Check sheet for the modelled part. Datum: model origin and axes. Units: mm. A direction names the side the tool comes from. Coordinates: 2 decimals unless noted, no trailing zeros. Loops run counter-clockwise (first coordinate to the right, second up) from the corner with the lowest first, then second, coordinate; pieces in that order, holes last.
```python
from build123d import *

# Parameters (mm, degrees)
BOSS_EXTRUDE9_DEPTH      = 3.5
BOSS_EXTRUDE9_DEPTH_BACK = 4
SKETCH16_W               = 8
SKETCH16_H               = 3.5
BOSS_EXTRUDE11_DEPTH     = 8
CHAMFER2_SIZE            = 1.5
CUT_EXTRUDE1_DEPTH       = 40.150823276
CUT_EXTRUDE1_DEPTH_BACK  = 40.150823276
SKETCH17_R               = 2.12


with BuildPart() as part:
    # Sketch14 → Boss-Extrude9 (new, two sides: drawn at the far end of the back side and taken through both)
    with BuildSketch(Plane(origin=(0, 0, 0), x_dir=(1, 0, 0), z_dir=(0, 1, 0)).offset(-BOSS_EXTRUDE9_DEPTH_BACK)):
        with BuildLine():
            Line((-4.172171186, -29.619968889), (7.827828814, -29.619968889))
            Line((7.827828814, -29.619968889), (7.827828814, -20.619968889))
            ThreePointArc((7.827828814, -20.619968889), (1.827828814, -14.619968889), (-4.172171186, -20.619968889))
            Line((-4.172171186, -20.619968889), (-4.172171186, -29.619968889))
        make_face()
    extrude(amount=BOSS_EXTRUDE9_DEPTH + BOSS_EXTRUDE9_DEPTH_BACK)

    # Sketch16 → Boss-Extrude11 (add)
    with BuildSketch(Plane.XY.offset(29.619968889)):
        with Locations((1.827828814, -0.25)):
            Rectangle(SKETCH16_W, SKETCH16_H)
    extrude(amount=BOSS_EXTRUDE11_DEPTH)

    # Chamfer2
    chamfer2_edges = [part.edges().sort_by_distance(p)[0] for p in [
        (1.827828814, -4, 14.619968889),
        (7.827828814, 3.5, 25.119968889),
        (1.827828814, 3.5, 14.619968889),
        (-4.172171186, -4, 25.119968889),
        (-4.172171186, 3.5, 25.119968889),
        (7.827828814, -4, 25.119968889),
    ]]
    chamfer(chamfer2_edges, length=CHAMFER2_SIZE)

    # Sketch17 → Cut-Extrude1 (cut, two sides: drawn at the far end of the back side and taken through both)
    with BuildSketch(Plane.XZ.offset(4).offset(-CUT_EXTRUDE1_DEPTH_BACK)):
        with Locations(Location((1.827828814, 25.119968889, 0), (0, 0, 270))):
            Circle(SKETCH17_R)
        with Locations(Location((1.827828814, 19.619968889, 0), (0, 0, 270))):
            Circle(SKETCH17_R)
    extrude(amount=CUT_EXTRUDE1_DEPTH + CUT_EXTRUDE1_DEPTH_BACK, mode=Mode.SUBTRACT)


solid = part.part
```
1) Set-up check for faces 4 (the flat face through (2, 1.5, 34)), 5 (the flat face through (-2.172, 0, 34)), 6 (the flat face through (2, -2, 34)): record each of +Z, -Z, +X, -X, +Y, -Y from which the full face is reachable in a straight line by a thin tool's end or side.
Answer sheet:
face 4: +Z, +X, -X, +Y
face 5: +Z, -X, +Y, -Y
face 6: +Z, +X, -X, -Y
2) Section check B-B on y = 0.5. Enter the section's corners in (x, z), plus the area to 3 significant figures.
Answer sheet:
outline: (-4.17, 20.62) arc R6 ccw to (7.83, 20.62) - (7.83, 29.62) - (5.83, 29.62) - (5.83, 37.62) - (-2.17, 37.62) - (-2.17, 29.62) - (-4.17, 29.62) - close; hole circle Ø4.24 at (1.83, 19.62); hole circle Ø4.24 at (1.83, 25.12)
area: 200 mm2
3) Depth check by flat-ended pin: pin 1 (1 mm diameter, centred on x = -1, z = 33.5, fed in from +Y); pin 2 (3 mm diameter, centred on y = 0.5, z = 34, fed in from +X); pin 3 (1 mm diameter, centred on y = -3, z = 32, fed in from -X); pin 4 (4 mm diameter, centred on x = 1, z = 33.5, fed in from -Y). Enter the tip coordinate at first touch or a pass-through.
Answer sheet:
pin 1: stops at y = 1.5
pin 2: stops at x = 5.83
pin 3: passes through
pin 4: stops at y = -2
4) Section check C-C on x = 1.25. Give the number of separate pieces and of enclosed holes in the cut face, plus the area to 3 significant figures.
Answer sheet:
separate pieces: 3
enclosed holes: 0
area: 76.8 mm2
5) Scan lines: line 1 (X direction, y = -0.75, z = 25); line 2 (Z direction, x = 1, y = 0.25); line 3 (Z direction, x = 2.75, y = 1.75). Record each from-to range of solid material in increasing order.
Answer sheet:
line 1: x = -4.17 to -0.29, 3.94 to 7.83
line 2: z = 14.68 to 17.67, 21.57 to 23.17, 27.07 to 37.62
line 3: z = 14.69 to 17.71, 21.53 to 23.21, 27.03 to 29.62
6) Mould release check, pull along X, two halves, no side actions. Record for faces 1 (the cylindrical face through (1.921, -0.197, 27.238)), 2 (the flat face through (2, 0, 37.62)), 3 (the flat face through (-3.43, 2.74, 25.06)): +X half, -X half, draft (parallel to the pull), parting line (faces both ways), or undercut.
Answer sheet:
face 1: undercut
face 2: draft
face 3: -X half
7) Section check A-A on z = 21.25. Enter the section's corners in (x, y), plus the area to 3 significant figures.
Answer sheet:
outline: (-4.17, -2.5) - (-2.67, -4) - (0.47, -4) - (0.47, 3.5) - (-2.67, 3.5) - (-4.17, 2) - close; (3.18, -4) - (6.33, -4) - (7.83, -2.5) - (7.83, 2) - (6.33, 3.5) - (3.18, 3.5) - close
area: 65.2 mm2
8) Section check D-D on z = 32.25. Enter the section's corners in (x, y), plus the area to 3 significant figures.
Answer sheet:
outline: (-2.17, -2) - (5.83, -2) - (5.83, 1.5) - (-2.17, 1.5) - close
area: 28.0 mm2
